from build123d import *

# Parameters (mm, degrees)
F0_W     = 50.8
F0_H     = 31.75
F1_DEPTH = 31.75
F3_DEPTH = 12.7
F5_DEPTH = 50.8
F7_DEPTH = 25.4


# Not quite as in the source:
# - a feature of the source that left no trace in its solid (it failed there, or was rolled back) is left out


with BuildPart() as f1:
    # F0 (on Right) → F1 (new body)
    with BuildSketch(Plane.YZ):
        with Locations((25.4, 15.875)):
            Rectangle(F0_W, F0_H)
    extrude(amount=F1_DEPTH)

    # F2 (on face) → F3 (cut)
    with BuildSketch(Plane.YZ.offset(31.75)):
        Polygon((19.05, 31.75), (50.8, 0), (50.8, 31.75), align=None)
    extrude(amount=-F3_DEPTH, mode=Mode.SUBTRACT)

    # F4 (on face) → F5 (cut)
    with BuildSketch(Plane.YZ.offset(19.05)):
        Polygon((19.05, 31.75), (34.925, 15.875), (38.1, 31.75), align=None)
    extrude(amount=-F5_DEPTH, mode=Mode.SUBTRACT)

    # F6 (on face) → F7 (cut)
    with BuildSketch(Plane.YZ.offset(19.05)):
        Polygon((38.1, 31.75), (34.925, 15.875), (50.8, 15.875), (50.8, 31.2204860245), align=None)
        Polygon((50.8, 31.75), (38.1, 31.75), (50.8, 31.2204860245), align=None)
    extrude(amount=-F7_DEPTH, mode=Mode.SUBTRACT)


solid = f1.part
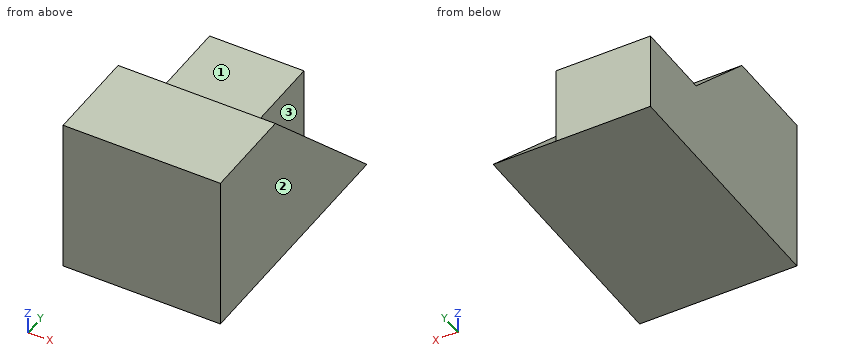
CAD build for the part. Positions are in the model's coordinates, mm. Face numbers are marked on the shaded views. A direction names the side the tool comes from. Coordinates: 2 decimals unless noted, no trailing zeros. Order: outer loops, then holes, each group sorted by start corner. A loop starts at its lowest first (then second) coordinate and runs counter-clockwise, first axis right, second up. Notation, with made-up numbers: (76.5, -31.5) -> (93.5, -31.5) arc R31 cw to (93.5, 0.5) -> close; hole circle Ø5 at (79.5, 55). An arc over 180 degrees is marked (long way). Answer in a Markdown table with one row per item.
1) Band-saw the part on D-D (y = 24.5). List the corners of the cut face in (x, z).
Check values:
| item | result |
|---|---|
| outline | (0, 0) -> (31.75, 0) -> (31.75, 26.3) -> (0, 26.3) -> close |
2) Band-saw the part on A-A (y = 39). List the corners of the cut face in (x, z) (3 decimals).
Check values:
| item | result |
|---|---|
| outline | (0, 0) -> (31.75, 0) -> (31.75, 11.8) -> (19.05, 11.8) -> (19.05, 15.875) -> (0, 15.875) -> close |
3) Drill centre lines: line 1 (Z direction, x = 3, y = 39.5) (3 decimals); line 2 (Z direction, x = 17, y = 25); line 3 (Y direction, x = 7.5, z = 20.5). Where is each one in solid material? Low to high.
Check values:
| item | result |
|---|---|
| line 1 | 0 to 15.875 |
| line 2 | 0 to 25.8 |
| line 3 | 0 to 30.3 |
4) Flat gauge pins, fed straight in: P1, Ø5, axis at x = 7.5, y = 40, coming from the +Z side (3 decimals); P2, Ø3, axis at x = 25.5, y = 42.5, coming from the +Z side; P3, Ø1.5, axis at x = 13, z = 20, coming from the +Y side. Where does each tip first touch, or does it go through?
Check values:
| item | result |
|---|---|
| P1 | z = 15.875 |
| P2 | z = 9.8 |
| P3 | y = 31.55 |
5) Band-saw the part on B-B (x = 6.5). List the corners of the cut face in (y, z) (3 decimals), and give its area (3 significant figures).
Check values:
| item | result |
|---|---|
| outline | (0, 0) -> (50.8, 0) -> (50.8, 15.875) -> (34.925, 15.875) -> (19.05, 31.75) -> (0, 31.75) -> close |
| area | 1,230 mm2 |
6) Which spindle directions (+Z, -Z, +X, -X, +Y, -Y) get a long thin tool onto all of the face, cutting with end or side? Do the marked faces 1, 2 and 3. Say none if no direction does.
Check values:
| item | result |
|---|---|
| face 1 | +Z, +X, -X, +Y |
| face 2 | +Z, -Z, +X, +Y, -Y |
| face 3 | +Z, +X, +Y |
7) Band-saw the part on C-C (z = 25). List the corners of the cut face in (x, y), and give its area (3 significant figures).
Check values:
| item | result |
|---|---|
| outline | (0, 0) -> (31.75, 0) -> (31.75, 25.8) -> (0, 25.8) -> close |
| area | 819 mm2 |
